Build history of the part. All positions in model axes, mm. A direction names the side the tool comes from. Give positions to 0.01 mm unless a question says otherwise; leave off trailing zeros. Loops run counter-clockwise (first coordinate to the right, second up) from the corner with the lowest first, then second, coordinate; pieces in that order, holes last. Notation, with made-up numbers: (-25, 71) -> (-7, 71) arc R31 cw to (-7, 96) -> close; hole circle Ø9 at (87, 44.25). An arc over 180 degrees is marked (long way). Answer in a Markdown table with one row per item. Add a question column.
from build123d import *

# Parameters (mm, degrees)
SKETCH1_W           = 24
SKETCH1_H           = 24
BOSS_EXTRUDE1_DEPTH = 165
FILLET1_R           = 10
SKETCH4_R           = 12
BOSS_EXTRUDE2_DEPTH = 1


with BuildPart() as part:
    # Sketch1 → Boss-Extrude1 (new body)
    with BuildSketch(Plane.XY):
        Rectangle(SKETCH1_W, SKETCH1_H)
    extrude(amount=BOSS_EXTRUDE1_DEPTH)

    # Sketch3 → Revolve1 (revolve)
    with BuildSketch(Plane(origin=(0, 0, 0), x_dir=(-1, 0, 0), z_dir=(0, -1, 0))):
        with BuildLine():
            Line((0, -165), (0, -180))
            ThreePointArc((0, -180), (9.604686356, -175.383749085), (12, -165))
            Line((12, -165), (0, -165))
        make_face()
    revolve(axis=Axis((0, 0, 165), (0, 0, 1)))

    # Fillet1
    fillet1_edges = [part.edges().sort_by_distance(p)[0] for p in [
        (12, -12, 82.5),
        (-12, -12, 82.5),
        (-12, 12, 82.5),
        (12, 12, 82.5),
    ]]
    fillet(fillet1_edges, radius=FILLET1_R)

    # Sketch4 → Boss-Extrude2 (add)
    with BuildSketch(Plane(origin=(0, 0, 0), x_dir=(-1, 0, 0), z_dir=(0, 0, -1))):
        Circle(SKETCH4_R)
    extrude(amount=BOSS_EXTRUDE2_DEPTH)


solid = part.part
(1) 3-axis set-ups, long thin cutter, end or side, ignore diameter. For faces 5 (the flat face through (-12, 0, 81)), 6 (the flat face through (-8.7, 8.7, 0)), 7 (the flat face through (0, -12, 81)), 8 (the flat face through (8.6, 8.7, 0)): which of +Z, -Z, +X, -X, +Y, -Y reach the whole face in a straight line?
(2) Flat gauge pins, fed straight in: pin 1 Ø1.2 at (y, z) = (-0.5, 86) entering from +X; pin 2 Ø2 at (x, z) = (-9, 158) entering from -Y; pin 3 Ø4.5 at (x, z) = (0.5, 113.5) entering from +Y. Where does each tip first touch, or does it go through?
(3) Saw through at B-B, the plane x = -7.75. List the corners of the cut face in (y, z), then the cut area to 3 significant figures.
(4) Saw through at A-A, the plane z = 14.5. List the corners of the cut face in (x, y), then the cut area to 3 significant figures.
(5) Wall check: line 1 along Y through (x, z) = (1, 142.5); line 2 along Z through (x, y) = (11, -6); line 3 along X through (y, z) = (-6.75, 120.5). Give the ranges that are in metal, low to high. Write a range as from..to.
(6) Two-plate mould, pull along Z, no slides. Class faces 1 (the flat face through (8.6, 8.7, 165)), 2 (the flat face through (12, 0, 81)), 3 (the flat face through (8.6, -8.6, 165)), 4 (the flat face through (-8.7, -8.6, 0)): released by +Z, released by -Z, zero draft, split by the parting line, or undercut.
(7) Saw through at C-C, the plane y = 8.5. List the corners of the cut face in (x, z), then the cut area to 3 significant figures.
Worked answers:
| question | item | result |
|---|---|---|
| 1 | face 5 | -Z, -X, +Y, -Y |
| 1 | face 6 | -Z, -X, +Y |
| 1 | face 7 | -Z, +X, -X, -Y |
| 1 | face 8 | -Z, +X, +Y |
| 2 | pin 1 | x = 12 |
| 2 | pin 2 | y = -10 |
| 2 | pin 3 | y = 12 |
| 3 | outline | (-10.18, 0) -> (-9.16, 0) -> (-9.16, -1) -> (9.16, -1) -> (9.16, 0) -> (10.18, 0) -> (10.18, 165) -> (9.16, 165) arc R9.55 ccw (long way) to (-9.16, 165) -> (-10.18, 165) -> close |
| 3 | area | 3,570 mm^2 |
| 4 | outline | (-12, -2) arc R10 ccw to (-2, -12) -> (2, -12) arc R10 ccw to (12, -2) -> (12, 2) arc R10 ccw to (2, 12) -> (-2, 12) arc R10 ccw to (-12, 2) -> close |
| 4 | area | 490 mm^2 |
| 5 | line 1 | -12..12 |
| 5 | line 2 | 0..165 |
| 5 | line 3 | -10.8..10.8 |
| 6 | face 1 | undercut |
| 6 | face 2 | zero draft |
| 6 | face 3 | undercut |
| 6 | face 4 | released by -Z |
| 7 | outline | (-9.6, 0) -> (-8.47, 0) -> (-8.47, -1) -> (8.47, -1) -> (8.47, 0) -> (9.6, 0) -> (9.6, 165) -> (8.47, 165) arc R8.89 ccw (long way) to (-8.47, 165) -> (-9.6, 165) -> close |
| 7 | area | 3,360 mm^2 |
